Autodesk Inventor part; units mm, degrees
ref_plane "YZ Plane" through (0, 0, 0) normal (1, 0, 0) x (0, 1, 0)
ref_plane "XZ Plane" through (0, 0, 0) normal (0, 1, 0) x (-1, 0, 0)
ref_plane "XY Plane" through (0, 0, 0) normal (0, 0, 1) x (1, 0, 0)
sketch "Sketch_1" plane through (0, 0, 0) normal (1, 0, 0) x (0, 1, 0)
  line L0 (0, 63.5) -> (0, 0)
  line L1 (0, 0) -> (63.5, 0)
  arc A0 (63.5, 0) -> (58.7248, 4.7752) centre (58.7248, 0) ccw
  line L2 (58.7248, 4.7752) -> (7.9502, 4.7752)
  arc A1 (4.7752, 7.9502) -> (7.9502, 4.7752) centre (7.9502, 7.9502) ccw
  line L3 (4.7752, 7.9502) -> (4.7752, 58.7248)
  arc A2 (4.7752, 58.7248) -> (0, 63.5) centre (0, 58.7248) ccw
extrude "Extrusion1" add sketch "Sketch_1" along normal mid plane 22.225
sketch "Sketch2" plane through (11.1125, 0, 0) normal (0, 0, -1) x (-1, 0, 0)
  point P0 (11.1125, 19.05)
hole "Hole1" at (0, 19.05, 0) direction (0, 0, 1) diameter 6.5278 depth 4.7752
sketch "Sketch3" plane through (11.1125, 0, 0) normal (0, 0, -1) x (-1, 0, 0)
  point P0 (11.1125, 44.45)
hole "Hole2" at (0, 44.45, 0) direction (0, 0, 1) diameter 6.5278 depth 4.7752
sketch "Sketch4" plane through (-11.1125, 0, 63.5) normal (0, -1, 0) x (1, 0, 0)
  point P0 (11.1125, -44.45)
hole "Hole3" at (0, 0, 19.05) direction (0, 1, 0) diameter 6.5278 depth 4.7752
sketch "Sketch5" plane through (-11.1125, 0, 63.5) normal (0, -1, 0) x (1, 0, 0)
  point P0 (11.1125, -19.05)
hole "Hole4" at (0, 0, 44.45) direction (0, 1, 0) diameter 6.5278 depth 4.7752
properties part number "4101"
Source: CAD feature listing. Evaluate the final solid. Frame: model axes, mm. A direction names the side the tool comes from. Coordinates: 2 decimals unless noted, no trailing zeros. Write each loop counter-clockwise with the first axis right and the second up, starting at its lowest first coordinate (ties: lowest second). Pieces come first, ordered by that corner, then holes. Notation, with made-up numbers: (-34, 76) - (-21, 76) arc R29 cw to (-21, 111) - close; hole circle Ø8 at (63, 33). An arc over 180 degrees is marked (long way). Answer as a JSON object with one key per item and string values.
Q1. Set-up query: faces 1 (the flat face through (11.112, 17, 4)), 2 (the flat face through (0, 4.775, 33)). Return all of +Z, -Z, +X, -X, +Y, -Y with unobstructed straight access to the full face (end or side cutting, diameter ignored); none if empty.
Ans:
{"face 1": "+Z, -Z, +X, +Y, -Y", "face 2": "+Z, +X, -X, +Y"}
Q2. Section query A-A, the plane x = 0. Output: boundary loops of the cut face in (y, z) (3 decimals).
Ans:
{"outline": "(0, 0) - (15.786, 0) - (15.786, 4.775) - (7.95, 4.775) arc R3.175 cw to (4.775, 7.95) - (4.775, 15.786) - (0, 15.786) - close; (0, 22.314) - (4.775, 22.314) - (4.775, 41.186) - (0, 41.186) - close; (0, 47.714) - (4.775, 47.714) - (4.775, 58.725) arc R4.775 ccw to (0, 63.5) - close; (22.314, 0) - (41.186, 0) - (41.186, 4.775) - (22.314, 4.775) - close; (47.714, 0) - (63.5, 0) arc R4.775 ccw to (58.725, 4.775) - (47.714, 4.775) - close"}
Q3. Draft query along Y for faces 3 (the cylindrical face through (-0.16, 3.34, 62.14)), 4 (the cylindrical face through (-0.14, 41.19, 2.42)), 5 (the cylindrical face through (1.25, 22.065, 2.421)), 6 (the flat face through (-11.112, 17, 4)). Return one class per face: released by +Y, released by -Y, zero draft, split by the parting line, or undercut.
Ans:
{"face 3": "released by +Y", "face 4": "undercut", "face 5": "undercut", "face 6": "zero draft"}
Q4. Section query D-D, the plane x = 7.5. Output: boundary loops of the cut face in (y, z) (3 decimals).
Ans:
{"outline": "(0, 0) - (63.5, 0) arc R4.775 ccw to (58.725, 4.775) - (7.95, 4.775) arc R3.175 cw to (4.775, 7.95) - (4.775, 58.725) arc R4.775 ccw to (0, 63.5) - close"}
Q5. Material intervals for line 1 (Z direction, x = 0, y = 2.45); line 2 (Z direction, x = 0, y = 2.2); line 3 (X direction, y = 3.4, z = 19.05), sorted ascending. Write a range as [from, to].
Ans:
{"line 1": "z = [0, 15.79], [22.31, 41.19], [47.71, 62.82]", "line 2": "z = [0, 15.79], [22.31, 41.19], [47.71, 62.96]", "line 3": "x = [-11.11, -3.26], [3.26, 11.11]"}
Q6. First-contact query: pin 1 Ø6.5 at (x, y) = (1.5, 38) entering from +Z; pin 2 Ø8.5 at (x, z) = (0, 44.45) entering from +Y. Flat tips, straight axial feed; report the tip coordinate or a pass-through.
Ans:
{"pin 1": "stops at z = 4.78", "pin 2": "stops at y = 4.78"}
Q7. Section query B-B, the plane z = 19.05. Output: boundary loops of the cut face in (x, y), plus the area to 3 significant figures.
Ans:
{"outline": "(-11.11, 0) - (-3.26, 0) - (-3.26, 4.78) - (-11.11, 4.78) - close; (3.26, 0) - (11.11, 0) - (11.11, 4.78) - (3.26, 4.78) - close", "area": "75.0 mm2"}
